```python
from build123d import *

# Parameters (mm, degrees)
KES_EKSTR_ZYON1_DEPTH = 5
PAH1_SIZE             = 1


with BuildPart() as part:
    # Çizim1 → Döndür1 (revolve)
    with BuildSketch(Plane.XY, mode=Mode.PRIVATE) as d_nd_r1_sk:
        with BuildLine():
            Line((0, 0), (-15, 0))
            Line((-15, 0), (-15, 3))
            Line((-15, 3), (-13, 5))
            ThreePointArc((-13, 5), (-13.688325627, 10.216881481), (-10, 13.97))
            Line((-10, 13.97), (-10, 14.97))
            ThreePointArc((-10, 14.97), (-9.414213562, 16.384213562), (-8, 16.97))
            ThreePointArc((-8, 16.97), (-6.26471847, 31.641681769), (-8.892788281, 46.18))
            ThreePointArc((-8.892788281, 46.18), (-10.800156882, 47.30566855), (-10.5, 49.5))
            Line((-10.5, 49.5), (-13, 52))
            Line((-13, 52), (-13, 70))
            Line((-13, 70), (-13, 75))
            Line((-13, 75), (-8.5, 75))
            Line((-8.5, 75), (-8.5, 70))
            Line((-8.5, 70), (-8.5, 67))
            Line((-8.5, 67), (0, 67))
            Line((0, 67), (0, 0))
        make_face()
    revolve(d_nd_r1_sk.sketch.rotate(Axis((0, 78.14654641, 0), (0, -1, 0)), 270), axis=Axis((0, 78.14654641, 0), (0, -1, 0)))

    # Çizim3 → Kes-Ekstrüzyon1 (cut)
    with BuildSketch(Plane(origin=(0, 75, 0), x_dir=(1, 0, 0), z_dir=(0, 1, 0))):
        with BuildLine():
            Line((-12.519984026, 3.5), (-7.745966692, 3.5))
            ThreePointArc((-7.745966692, 3.5), (-6.01040764, 6.01040764), (-3.5, 7.745966692))
            Line((-3.5, 7.745966692), (-3.5, 12.519984026))
            ThreePointArc((-3.5, 12.519984026), (-9.192388155, 9.192388155), (-12.519984026, 3.5))
        make_face()
        with BuildLine():
            Line((-12.519984026, -3.5), (-7.745966692, -3.5))
            ThreePointArc((-7.745966692, -3.5), (-6.01040764, -6.01040764), (-3.5, -7.745966692))
            Line((-3.5, -7.745966692), (-3.5, -12.519984026))
            ThreePointArc((-3.5, -12.519984026), (-9.192388155, -9.192388155), (-12.519984026, -3.5))
        make_face()
        with BuildLine():
            Line((7.745966692, -3.5), (12.519984026, -3.5))
            ThreePointArc((12.519984026, -3.5), (9.192388155, -9.192388155), (3.5, -12.519984026))
            Line((3.5, -12.519984026), (3.5, -7.745966692))
            ThreePointArc((3.5, -7.745966692), (6.01040764, -6.01040764), (7.745966692, -3.5))
        make_face()
        with BuildLine():
            Line((12.519984026, 3.5), (7.745966692, 3.5))
            ThreePointArc((7.745966692, 3.5), (6.01040764, 6.01040764), (3.5, 7.745966692))
            Line((3.5, 7.745966692), (3.5, 12.519984026))
            ThreePointArc((3.5, 12.519984026), (9.192388155, 9.192388155), (12.519984026, 3.5))
        make_face()
    extrude(amount=-KES_EKSTR_ZYON1_DEPTH, mode=Mode.SUBTRACT)

    # Pah1
    pah1_edges = [part.edges().sort_by_distance(p)[0] for p in [
        (13, 75, 0),
        (-13, 75, 0),
        (-1.766381565, 75, 12.879436951),
        (8.5, 75, 0),
        (0, 75, -8.5),
        (-8.5, 75, 0),
        (-1.790151267, 75, 8.309353672),
    ]]
    chamfer(pah1_edges, length=PAH1_SIZE)


solid = part.part
```
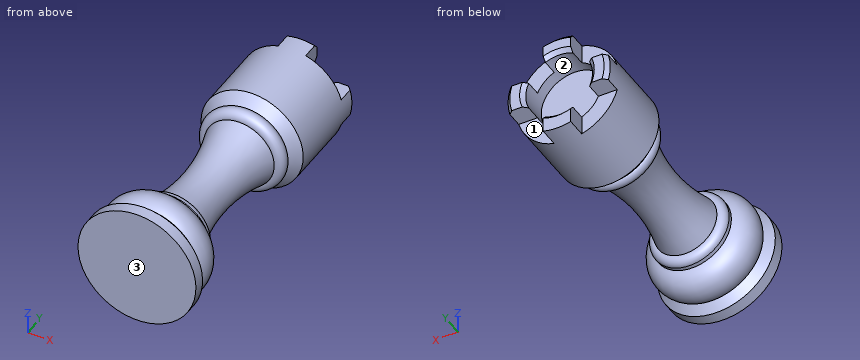
Read the model definition and answer for the solid it produces. Units are mm, in the model's axes. Face numbers are marked on the shaded views. A direction names the side the tool comes from. Give positions to 0.01 mm unless a question says otherwise; leave off trailing zeros. Loops run counter-clockwise (first coordinate to the right, second up) from the corner with the lowest first, then second, coordinate; pieces in that order, holes last.
Item 1: The part is cut by section C-C (y = 55). Write down the section's boundary in (x, z), and give its area (3 significant figures).
Item 2: Find the intervals of material crossed by line 1 along X through (y, z) = (70, 0); line 2 along Y through (x, z) = (7.25, 8); line 3 along Y through (x, z) = (-3.75, 1), in increasing order.
Item 3: The part is cut by section A-A (z = 0). Write down the section's boundary in (x, y), and give its area (3 significant figures).
Item 4: The part is cut by section D-D (y = 44.5). Write down the section's boundary in (x, z).
Item 5: Each of these flat-tipped pins is pushed along its axis until it touches: pin 1 Ø5.5 at (y, z) = (73.5, -9.5) entering from -X; pin 2 Ø8 at (y, z) = (54.5, 8.5) entering from -X; pin 3 Ø3 at (x, y) = (-0.5, 36.5) entering from -Z. Where does it stop, or does it pass through?
Item 6: For the marked faces 1, 2 and 3, determine the directions among +Z, -Z, +X, -X, +Y, -Y from which every point of the face is accessible in a straight line to the end or side of a thin tool.
Item 7: The part is cut by section B-B (x = 0). Write down the section's boundary in (y, z), and give its area (3 significant figures).
Taken from the geometry:
1. outline: circle Ø26 at (0, 0)
1. area: 531 mm2
2. line 1: x = -13 to -8.5, 8.5 to 13
2. line 2: y = 0 to 13.62, 47.3 to 49.06, 49.8 to 70
2. line 3: y = 0 to 67
3. outline: (-15, 0) - (15, 0) - (15, 3) - (13, 5) arc R6 ccw to (10, 13.97) - (10, 14.97) arc R2 ccw to (8, 16.97) arc R50 cw to (8.89, 46.18) arc R2 ccw to (10.5, 49.5) - (13, 52) - (13, 74) - (12, 75) - (9.5, 75) - (8.5, 74) - (8.5, 67) - (-8.5, 67) - (-8.5, 74) - (-9.5, 75) - (-12, 75) - (-13, 74) - (-13, 52) - (-10.5, 49.5) arc R2 ccw to (-8.89, 46.18) arc R50 cw to (-8, 16.97) arc R2 ccw to (-10, 14.97) - (-10, 13.97) arc R6 ccw to (-13, 5) - (-15, 3) - close
3. area: 1,440 mm2
4. outline: circle Ø16.71 at (0, 0)
5. pin 1: stops at x = -3.5
5. pin 2: stops at x = -12.2
5. pin 3: stops at z = -6.86
6. face 1: -Z, +X, +Y
6. face 2: +Y
6. face 3: +Z, -Z, +X, -X, -Y
7. outline: (0, -15) - (3, -15) - (5, -13) arc R6 ccw to (13.97, -10) - (14.97, -10) arc R2 ccw to (16.97, -8) arc R50 cw to (46.18, -8.89) arc R2 ccw to (49.5, -10.5) - (52, -13) - (75, -13) - (75, -9.5) - (74, -8.5) - (67, -8.5) - (67, 8.5) - (74, 8.5) - (75, 9.5) - (75, 12) - (74, 13) - (52, 13) - (49.5, 10.5) arc R2 ccw to (46.18, 8.89) arc R50 cw to (16.97, 8) arc R2 ccw to (14.97, 10) - (13.97, 10) arc R6 ccw to (5, 13) - (3, 15) - (0, 15) - close
7. area: 1,440 mm2
